```python
from build123d import *

# Parameters (mm, degrees)
CROQUIS1_R              = 2.25
SALIENTE_EXTRUIR1_DEPTH = 2
REDONDEO1_R             = 10


with BuildPart() as part:
    # Croquis1 → Saliente-Extruir1 (new body)
    with BuildSketch(Plane.XY):
        with BuildLine():
            Line((-85, 0), (85, 0))
            Line((85, 0), (85, 25))
            Line((85, 25), (51.567231643, 86.5))
            Line((51.567231643, 86.5), (30, 90.5))
            Line((30, 90.5), (17, 77.5))
            ThreePointArc((17, 77.5), (8.593451955, 79.385473293), (0, 80))
            ThreePointArc((0, 80), (-8.593451955, 79.385473293), (-17, 77.5))
            Line((-17, 77.5), (-30, 90.5))
            Line((-30, 90.5), (-51.567231643, 86.5))
            Line((-51.567231643, 86.5), (-85, 25))
            Line((-85, 25), (-85, 0))
        make_face()
        with Locations((-60, 37.5)):
            Circle(CROQUIS1_R, mode=Mode.SUBTRACT)
        with Locations((60, 37.5)):
            Circle(CROQUIS1_R, mode=Mode.SUBTRACT)
    extrude(amount=SALIENTE_EXTRUIR1_DEPTH)

    # Redondeo1
    redondeo1_edges = [part.edges().sort_by_distance(p)[0] for p in [
        (-85, 25, 1),
        (-51.567231643, 86.5, 1),
        (-30, 90.5, 1),
        (-17, 77.5, 1),
        (17, 77.5, 1),
        (30, 90.5, 1),
        (51.567231643, 86.5, 1),
        (85, 25, 1),
    ]]
    fillet(redondeo1_edges, radius=REDONDEO1_R)


solid = part.part
```
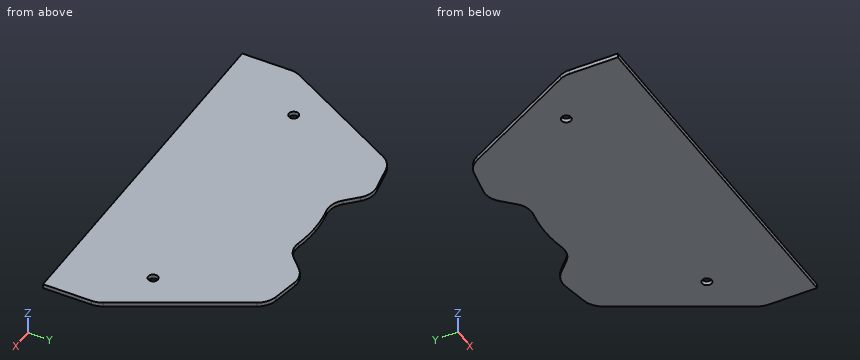
Work out the finished part from the listing and answer in its coordinate system (mm). Coordinates: 2 decimals unless noted, no trailing zeros. Order: outer loops, then holes, each group sorted by start corner. A loop starts at its lowest first (then second) coordinate and runs counter-clockwise, first axis right, second up. Notation, with made-up numbers: M -24.5,39.25 L 0.5,39.25 A16 cw 0.5,65.25 Z; hole C -15,-6.5 d11. An arc over 180 degrees is marked long. Use CSV: the item, a comma, the result in double quotes.
1) Section C-C on x = 17 is taken. Write down the section's boundary in (y, z).
Worked out:
outline,"M 0,0 L 79.07,0 L 79.07,2 L 0,2 Z"
2) Section B-B on x = -60 is taken. Write down the section's boundary in (y, z), plus the area to 3 significant figures.
Worked out:
outline,"M 0,0 L 35.25,0 L 35.25,2 L 0,2 Z; M 39.75,0 L 70.99,0 L 70.99,2 L 39.75,2 Z"
area,"133 mm^2"
3) Consider line 1 (Y direction, x = 19, z = 1.05); line 2 (Y direction, x = -60, z = 1.5); line 3 (X direction, y = 83, z = 0.85). Determine where each line is inside the solid, lowest interval first. Write a range as [from, to].
Worked out:
line 1,"y = [0, 79.96]"
line 2,"y = [0, 35.25], [39.75, 70.99]"
line 3,"x = [-53.43, -22.5], [22.5, 53.43]"
4) Section D-D on y = 54 is taken. Write down the section's boundary in (x, z), plus the area to 3 significant figures.
Worked out:
outline,"M -69.23,0 L 69.23,0 L 69.23,2 L -69.23,2 Z"
area,"277 mm^2"
5) Section A-A on z = 1.4 is taken. Write down the section's boundary in (x, y), plus the area to 3 significant figures.
Worked out:
outline,"M -85,0 L 85,0 L 85,22.46 A10 ccw 83.79,27.23 L 53.84,82.31 A10 ccw 46.88,87.37 L 35.17,89.54 A10 ccw 26.28,86.78 L 21.02,81.52 A10 cw 11.92,78.8 A57.78 ccw 0,80 A57.78 ccw -11.92,78.8 A10 cw -21.02,81.52 L -26.28,86.78 A10 ccw -35.17,89.54 L -46.88,87.37 A10 ccw -53.84,82.31 L -83.79,27.23 A10 ccw -85,22.46 Z; hole C -60,37.5 d4.5; hole C 60,37.5 d4.5"
area,"12,400 mm^2"
